```python
from build123d import *

# Parameters (mm, degrees)
SKETCH2_W           = 290
SKETCH2_H           = 30
SKETCH2_R           = 8
SKETCH2_W_2         = 30
SKETCH2_H_2         = 90
BOSS_EXTRUDE5_DEPTH = 5


with BuildPart() as part:
    # Sketch2 → Boss-Extrude5 (new body)
    # profile 1 of 2: a face of its own
    with BuildSketch(Plane(origin=(0, 0, 0), x_dir=(1, 0, 0), z_dir=(0, 1, 0))):
        with Locations((145, -15)):
            Rectangle(SKETCH2_W, SKETCH2_H)
        with Locations(Location((15, -15, 0), (0, 0, 270))):
            Circle(SKETCH2_R, mode=Mode.SUBTRACT)
        with Locations(Location((275, -15, 0), (0, 0, 270))):
            Circle(SKETCH2_R, mode=Mode.SUBTRACT)
        with Locations(Location((75, -15, 0), (0, 0, 270))):
            Circle(SKETCH2_R, mode=Mode.SUBTRACT)
    # profile 2 of 2: a face of its own
    with BuildSketch(Plane(origin=(0, 0, 0), x_dir=(1, 0, 0), z_dir=(0, 1, 0))):
        with Locations((175, 25)):
            Rectangle(SKETCH2_W_2, SKETCH2_H_2)
        with Locations(Location((175, 55, 0), (0, 0, 270))):
            Circle(SKETCH2_R, mode=Mode.SUBTRACT)
    extrude(amount=BOSS_EXTRUDE5_DEPTH)


solid = part.part
```
Could you check a few things on this model? Use its own coordinates, in mm. A direction names the side the tool comes from. Give positions to 0.01 mm unless a question says otherwise; leave off trailing zeros. Write each loop counter-clockwise with the first axis right and the second up, starting at its lowest first coordinate (ties: lowest second). Pieces come first, ordered by that corner, then holes. Notation, with made-up numbers: (9, 78) - (59, 78) arc R27 ccw to (59, 110) - close; hole circle Ø11 at (-11.5, 83). An arc over 180 degrees is marked (long way). One line per item, written item: value. Start each with the question number.
Item 1: Please list where these lines run through material, in increasing order: line 1 (X direction, y = 2.5, z = 15); line 2 (X direction, y = 2.6, z = -55); line 3 (X direction, y = 2.75, z = -14). Write a range as from..to.
Item 2: Imagine slicing it at D-D, the plane z = -55. List the corners of the cut face in (x, y) for me.
Item 3: Imagine slicing it at C-C, the plane y = 4.05. List the corners of the cut face in (x, z) for me, and give its area (4 significant figures).
Item 4: Imagine slicing it at A-A, the plane x = 175. List the corners of the cut face in (y, z) for me, and give its area (3 significant figures).
Item 5: Imagine slicing it at B-B, the plane z = 15. List the corners of the cut face in (x, y) for me.
Item 6: I'm going to push flat-ended pins straight in: pin 1 (2.5 mm diameter, centred on x = 220.5, y = 2, fed in from -Z); pin 2 (2.5 mm diameter, centred on y = 3.5, z = -38.5, fed in from -X); pin 3 (2 mm diameter, centred on y = 1.5, z = -49, fed in from +X). Where does each tip first touch, or does it pass through?
Item 7: If we mould it in two halves opening along X, with no side actions, what happens to faces 4 (the face through (282.932, 2.465, 13.959)), 5 (the face through (155, 0, 6)), 6 (the face through (0, 2, 15))? For each: +X half, -X half, draft (parallel to the pull), parting line (faces both ways), or undercut.
Item 8: Which directions (+Z, -Z, +X, -X, +Y, -Y) give clear straight access to the entire face, cutting with the end or side of a thin tool? Please do faces 1 (the face through (160, 2, -35)), 2 (the face through (190, 2, -35)), 3 (the face through (82.932, 2.465, 13.959)).
Geometry says:
1. line 1: 0..7, 23..67, 83..267, 283..290
1. line 2: 160..167, 183..190
1. line 3: 160..190
2. outline: (160, 0) - (167, 0) - (167, 5) - (160, 5) - close; (183, 0) - (190, 0) - (190, 5) - (183, 5) - close
3. outline: (0, 0) - (160, 0) - (160, -70) - (190, -70) - (190, 0) - (290, 0) - (290, 30) - (0, 30) - close; hole circle Ø16 at (15, 15); hole circle Ø16 at (75, 15); hole circle Ø16 at (175, -55); hole circle Ø16 at (275, 15)
3. area: 10,000 mm^2
4. outline: (0, -70) - (5, -70) - (5, -63) - (0, -63) - close; (0, -47) - (5, -47) - (5, 30) - (0, 30) - close
4. area: 420 mm^2
5. outline: (0, 0) - (7, 0) - (7, 5) - (0, 5) - close; (23, 0) - (67, 0) - (67, 5) - (23, 5) - close; (83, 0) - (267, 0) - (267, 5) - (83, 5) - close; (283, 0) - (290, 0) - (290, 5) - (283, 5) - close
6. pin 1: z = 0
6. pin 2: x = 160
6. pin 3: x = 190
7. face 4: undercut
7. face 5: draft
7. face 6: -X half
8. face 1: -Z, -X, +Y, -Y
8. face 2: -Z, +X, +Y, -Y
8. face 3: +Y, -Y
